Here's how the part is built. I have some questions about the finished solid (model axes, mm). Face numbers are marked on the shaded views. Give positions to 0.01 mm unless a question says otherwise; leave off trailing zeros. Write each loop counter-clockwise with the first axis right and the second up, starting at its lowest first coordinate (ties: lowest second). Pieces come first, ordered by that corner, then holes. Notation, with made-up numbers: M 72,48.25 L 118,48.25 A15 cw 118,68.25 Z; hole C 85.5,39 d5. An arc over 180 degrees is marked long. Use one line per item in the form item = value. Start each with the question number.
from build123d import *

# Parameters (mm, degrees)
SKETCH1_R               = 76.2
BOSS_EXTRUDE1_DEPTH     = 9.525
CIRPATTERN6_COUNT       = 3
F_3_8_CLEARANCE_HOLE1_D = 9.8044
F_1_4_CLEARANCE_HOLE1_D = 6.5278


with BuildPart() as part:
    # Sketch1 → Boss-Extrude1 (new body)
    with BuildSketch(Plane(origin=(0, 0, 0), x_dir=(1, 0, 0), z_dir=(0, 1, 0))):
        with Locations(Location((0, 0, 0), (0, 0, 90))):
            Circle(SKETCH1_R)
    extrude(amount=BOSS_EXTRUDE1_DEPTH)

    # Sketch5 → Cut-Revolve1 (revolve, cut)
    with BuildSketch(Plane.XY, mode=Mode.PRIVATE) as cut_revolve1_sk:
        Polygon((0, 0), (0, 9.525), (15.552216058, 9.525), (13, 0), align=None)
    revolve(cut_revolve1_sk.sketch.rotate(Axis((0, 0, 0), (0, 1, 0)), 90), axis=Axis((0, 0, 0), (0, 1, 0)), mode=Mode.SUBTRACT)

    # Sketch15 → 1/4 NPT Tapped Hole1 (revolve, cut)
    with BuildSketch(Plane(origin=(33.011727721, 9.525, -27.700128555), x_dir=(0, 0, 1), z_dir=(1, 0, 0))):
        Polygon((0, 0), (0, 9.525), (5.5626, 9.525), (5.5626, 10.0203), (6.557978799, 10.0203), (6.858, 0), align=None)
    f_1_4_npt_tapped_hole1 = revolve(axis=Axis((33.011727721, 15.875, -27.700128555), (0, -1, 0)), mode=Mode.SUBTRACT)

    # CirPattern6: 1/4 NPT Tapped Hole1 ×3 about axis
    cirpattern6_axis = Axis((0, 0, 0), (0, 1, 0))
    for i in range(1, CIRPATTERN6_COUNT):
        add(f_1_4_npt_tapped_hole1.rotate(cirpattern6_axis, i * 360 / CIRPATTERN6_COUNT), mode=Mode.SUBTRACT)

    # 3/8 Clearance Hole1 (through all)
    with Locations(Plane(origin=(0, 9.525, 0), x_dir=(1, 0, 0), z_dir=(0, 1, 0))):
        with Locations((60.207217661, 25.013604371), (60.257374801, -24.888494705), (24.885638551, 60.264250563), (-25.016460514, 60.214093421), (-60.267106699, 24.892514335), (-60.216949569, -25.009584719), (-24.895370482, -60.260230921), (25.006728592, -60.210073801)):
            Hole(F_3_8_CLEARANCE_HOLE1_D / 2)

    # 1/4 Clearance Hole1 (through all)
    with Locations(Plane(origin=(0, 9.525, 0), x_dir=(1, 0, 0), z_dir=(0, 1, 0))):
        with Locations((-20.240427094, 15.531025958), (20.240427094, -15.531025958), (-23.570476573, -9.763211068), (23.570476573, 9.763211068)):
            Hole(F_1_4_CLEARANCE_HOLE1_D / 2)


solid = part.part
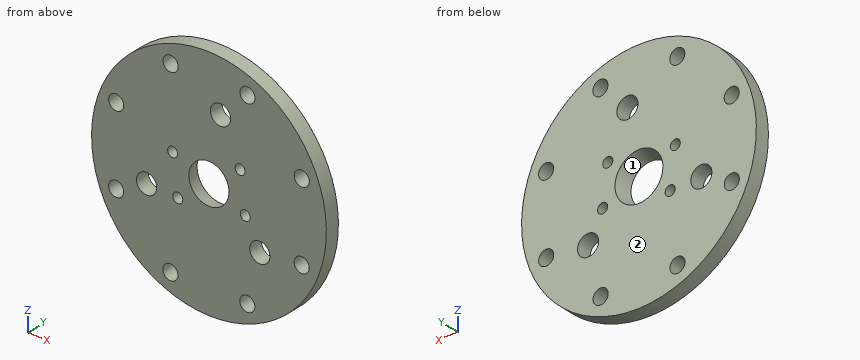
1) Suppose I cut it at D-D, the plane z = -52.5. List the corners of the cut face in (x, y) for me (3 decimals), and give its area (3 significant figures).
2) Please list where these lines run through material, in increasing order: line 1 (Z direction, x = 10.5, y = 7.25); line 2 (X direction, y = 1, z = 21); line 3 (Z direction, x = -22, y = 8.25).
3) Suppose I cut it at C-C, the plane x = 47. List the corners of the cut face in (y, z) for me (3 decimals).
4) Will these pins go through, and if not, where does the flat tip stop? P1, Ø12.5, axis at x = 24.89, z = -60.26, coming from the -Y side; P2, Ø2, axis at x = 1.5, y = 5.5, coming from the +Z side; P3, Ø1.5, axis at y = 6, z = -59, coming from the -X side; P4, Ø2, axis at y = 4.5, z = 39.5, coming from the -X side.
5) Suppose I cut it at B-B, the plane x = 63. List the corners of the cut face in (y, z) for me (1 decimal), and give its area (3 significant figures).
6) Suppose I cut it at A-A, the plane z = 0. List the corners of the cut face in (x, y) for me (3 decimals).
7) Thinking about a two-plate mould opening in Z: for the marked faces 1 and 2, which applies, released by +Z, released by -Z, zero draft, split by the parting line, or undercut?
Checks:
q1.outline = M -55.229,0 L 55.229,0 L 55.229,9.525 L -55.229,9.525 Z
q1.area = 1,050 mm^2
q2.line_1 = -75.47 to -10.63, 10.63 to 36.36, 48.52 to 75.47
q2.line_2 = -73.25 to -63.04, -57.4 to 57.27, 63.24 to 73.25
q2.line_3 = -72.96 to -64.08, -56.35 to -18.28, -12.78 to 6.9, 12.62 to 56.3, 64.22 to 72.96
q3.outline = M 0,-59.979 L 9.525,-59.979 L 9.525,59.979 L 0,59.979 Z
q4.P1 = 0
q4.P2 = 76.2
q4.P3 = -49.13
q4.P4 = -65.76
q5.outline = M 0,-42.9 L 9.5,-42.9 L 9.5,-29 L 0,-29 Z; M 0,-21 L 9.5,-21 L 9.5,20.8 L 0,20.8 Z; M 0,29 L 9.5,29 L 9.5,42.9 L 0,42.9 Z
q5.area = 662 mm^2
q6.outline = M -76.2,0 L -13,0 L -15.552,9.525 L -76.2,9.525 Z; M 13,0 L 76.2,0 L 76.2,9.525 L 15.552,9.525 Z
q7.face_1 = undercut
q7.face_2 = zero draft
